Verification items for the finished model (mm, model axes). Face numbers are marked on the shaded views. A direction names the side the tool comes from. Coordinates: 2 decimals unless noted, no trailing zeros. Order: outer loops, then holes, each group sorted by start corner. A loop starts at its lowest first (then second) coordinate and runs counter-clockwise, first axis right, second up. Notation, with made-up numbers: M 72.25,86.25 L 102.25,86.25 A9 ccw 102.25,103.25 Z; hole C 24.25,25 d8. An arc over 180 degrees is marked long. Return JSON: item names as keys, results as strings. Group by question number.
Q1. Section check D-D, the plane y = 18.5. Enter the section's corners in (x, z), then the cut area to 3 significant figures.
Q2. Section check C-C, the plane y = 10.5. Enter the section's corners in (x, z), then the cut area to 3 significant figures.
Q3. Go/stop test with flat-tipped pins: pin 1 Ø5 at (y, z) = (15.5, 9) entering from +X; pin 2 Ø9 at (x, z) = (-19, 7.5) entering from +Y; pin 3 Ø6 at (x, y) = (0, -5) entering from +Z; pin 4 Ø1.8 at (x, y) = (0, -5) entering from +Z. Record where each tip stops, or that it passes through.
Q4. Access from +Z, -Z, +X, -X, +Y, -Y to the whole of each face (thin tool, end or side, straight path). Record for the marked faces 4, 5, 6 and 7.
Q5. Mould release check, pull along Z, two halves, no side actions. Record for the marked faces 1, 2 and 3: pulls with the +Z half, pulls with the -Z half, needs draft (parallel to the pull), parting line crosses it, or undercut.
Q6. Thickness scan on probe 1 along Z at (x, y) = (-6, -26); probe 2 along Z at (x, y) = (19, -10); probe 3 along X at (y, z) = (-27, 10.5). Record the ranges inside material, lowest first.
Q7. Section check B-B, the plane x = 19. Enter the section's corners in (y, z), then the cut area to 3 significant figures.
Q8. Section check A-A, the plane z = 7.5. Count the separate pieces of the cut face and the enclosed holes in it, then the cut area to 3 significant figures.
from build123d import *

# Parameters (mm, degrees)
BOSS_EXTRUDE1_DEPTH = 15
CUT_EXTRUDE1_REACH  = 17
CUT_EXTRUDE2_DEPTH  = 1.5
CUT_EXTRUDE3_REACH  = 15.5
SKETCH4_R           = 1.5
SKETCH5_R           = 2.5
CUT_EXTRUDE4_DEPTH  = 12
SKETCH6_R           = 0.48
BOSS_EXTRUDE2_DEPTH = 1.5
CUT_EXTRUDE5_REACH  = 57
SKETCH7_R           = 2.25
SKETCH8_R           = 5.54
CUT_EXTRUDE6_DEPTH  = 21
CUT_EXTRUDE7_REACH  = 57
SKETCH9_W           = 24
SKETCH9_H           = 7


with BuildPart() as part:
    # Sketch1 → Boss-Extrude1 (new body)
    with BuildSketch(Plane.XY):
        with BuildLine():
            Line((-25, 0), (-25, -30))
            Line((-25, -30), (25, -30))
            Line((25, -30), (25, 0))
            ThreePointArc((25, 0), (0, 25), (-25, 0))
        make_face()
    extrude(amount=BOSS_EXTRUDE1_DEPTH)

    # Sketch2 → Cut-Extrude1 (cut, up to next)
    with BuildSketch(Plane.XY.offset(15), mode=Mode.PRIVATE) as cut_extrude1_sk1:
        with BuildLine():
            Line((-15, -5), (-11.25, -5))
            ThreePointArc((-11.25, -5), (4.305188614, -15.393644741), (7.954951288, 2.954951288))
            Line((7.954951288, 2.954951288), (10.606601718, 5.606601718))
            ThreePointArc((10.606601718, 5.606601718), (5.740251485, -18.858192988), (-15, -5))
        make_face()
    cut_extrude1_tool1 = extrude(cut_extrude1_sk1.sketch, amount=-CUT_EXTRUDE1_REACH, mode=Mode.PRIVATE) & part.part
    add(cut_extrude1_tool1.solids().sort_by_distance((9.559676, 4.001877, 15))[0], mode=Mode.SUBTRACT)

    # Sketch3 → Cut-Extrude2 (cut)
    with BuildSketch(Plane.XY.offset(15)):
        with BuildLine():
            Line((-14.191020378, 1.753883373), (-0.462045472, -1.78301166))
            ThreePointArc((-0.462045472, -1.78301166), (3.054001018, -6.111565466), (-2.421787612, -7.167358937))
            Line((-2.421787612, -7.167358937), (-15.212264853, -1.05196276))
            ThreePointArc((-15.212264853, -1.05196276), (-15.974774553, 0.814342437), (-14.191020378, 1.753883373))
        make_face()
    extrude(amount=-CUT_EXTRUDE2_DEPTH, mode=Mode.SUBTRACT)

    # Sketch4 → Cut-Extrude3 (cut, up to next)
    with BuildSketch(Plane.XY.offset(13.5), mode=Mode.PRIVATE) as cut_extrude3_sk1:
        with Locations((0, -5)):
            Circle(SKETCH4_R)
    cut_extrude3_tool1 = extrude(cut_extrude3_sk1.sketch, amount=-CUT_EXTRUDE3_REACH, mode=Mode.PRIVATE) & part.part
    add(cut_extrude3_tool1.solids().sort_by_distance((0, -5, 13.5))[0], mode=Mode.SUBTRACT)

    # Sketch5 → Cut-Extrude4 (cut)
    with BuildSketch(Plane(origin=(0, 0, 0), x_dir=(-1, 0, 0), z_dir=(0, 0, -1))):
        with Locations((0, -5)):
            Circle(SKETCH5_R)
    extrude(amount=-CUT_EXTRUDE4_DEPTH, mode=Mode.SUBTRACT)

    # Sketch6 → Boss-Extrude2 (add)
    with BuildSketch(Plane.XY.offset(13.5)):
        with Locations((-14.565235622, 0.301312222)):
            Circle(SKETCH6_R)
        with Locations((-12.497911856, -0.451132094)):
            Circle(SKETCH6_R)
        with Locations((-10.430588091, -1.203576409)):
            Circle(SKETCH6_R)
        with Locations((-8.363264325, -1.956020724)):
            Circle(SKETCH6_R)
        with Locations((-6.295940559, -2.70846504)):
            Circle(SKETCH6_R)
        with Locations((-4.228616794, -3.460909355)):
            Circle(SKETCH6_R)
    extrude(amount=BOSS_EXTRUDE2_DEPTH)

    # Sketch7 → Cut-Extrude5 (cut, up to next)
    with BuildSketch(Plane.XZ.offset(30), mode=Mode.PRIVATE) as cut_extrude5_sk1:
        with Locations((-19, 7.5)):
            Circle(SKETCH7_R)
    cut_extrude5_tool1 = extrude(cut_extrude5_sk1.sketch, amount=-CUT_EXTRUDE5_REACH, mode=Mode.PRIVATE) & part.part
    add(cut_extrude5_tool1.solids().sort_by_distance((-19, -30, 7.5))[0], mode=Mode.SUBTRACT)
    # Sketch7 → Cut-Extrude5 (cut, up to next)
    with BuildSketch(Plane.XZ.offset(30), mode=Mode.PRIVATE) as cut_extrude5_sk2:
        with Locations((19, 7.5)):
            Circle(SKETCH7_R)
    cut_extrude5_tool2 = extrude(cut_extrude5_sk2.sketch, amount=-CUT_EXTRUDE5_REACH, mode=Mode.PRIVATE) & part.part
    add(cut_extrude5_tool2.solids().sort_by_distance((19, -30, 7.5))[0], mode=Mode.SUBTRACT)

    # Sketch8 → Cut-Extrude6 (cut)
    with BuildSketch(Plane(origin=(0, 23.467134405, 0), x_dir=(1, 0, 0), z_dir=(0, 1, 0))):
        with Locations((-19, -7.5)):
            Circle(SKETCH8_R)
        with Locations((19, -7.5)):
            Circle(SKETCH8_R)
    extrude(amount=-CUT_EXTRUDE6_DEPTH, mode=Mode.SUBTRACT)

    # Sketch9 → Cut-Extrude7 (cut, up to next)
    with BuildSketch(Plane.XZ.offset(30), mode=Mode.PRIVATE) as cut_extrude7_sk1:
        with Locations((0, 7.5)):
            Rectangle(SKETCH9_W, SKETCH9_H)
    cut_extrude7_tool1 = extrude(cut_extrude7_sk1.sketch, amount=-CUT_EXTRUDE7_REACH, mode=Mode.PRIVATE) & part.part
    add(cut_extrude7_tool1.solids().sort_by_distance((0, -30, 7.5))[0], mode=Mode.SUBTRACT)


solid = part.part
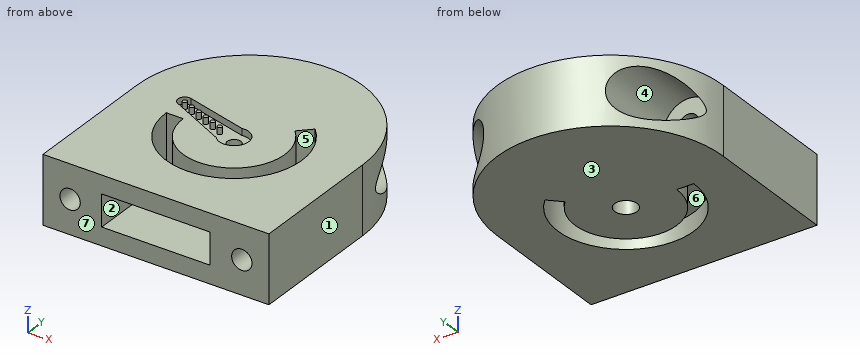
Numbers:
{
 "1": {"outline": "M -16.82,0 L 16.82,0 L 16.82,2.41 A5.54 cw 16.82,12.59 L 16.82,15 L -16.82,15 L -16.82,12.59 A5.54 cw -16.82,2.41 Z", "area": "455 mm2"},
 "2": {"outline": "M -22.69,0 L 22.69,0 L 22.69,3.37 A5.54 cw long 22.69,11.63 L 22.69,15 L -22.69,15 L -22.69,11.63 A5.54 cw long -22.69,3.37 Z", "area": "509 mm2"},
 "3": {"pin 1": "stops at x = 15.17", "pin 2": "stops at y = 2.47", "pin 3": "stops at z = 13.5", "pin 4": "passes through"},
 "4": {"face 4": "+Y", "face 5": "+Z, -Z", "face 6": "-Y", "face 7": "+Z, -Z, +X, -X, -Y"},
 "5": {"face 1": "needs draft", "face 2": "undercut", "face 3": "pulls with the -Z half"},
 "6": {"probe 1": "z = 0 to 4, 11 to 15", "probe 2": "z = 0 to 5.25, 9.75 to 15", "probe 3": "x = -25 to -12, 12 to 25"},
 "7": {"outline": "M -30,0 L 16.25,0 L 16.25,1.96 L 2.47,1.96 L 2.47,5.25 L -30,5.25 Z; M -30,9.75 L 2.47,9.75 L 2.47,13.04 L 16.25,13.04 L 16.25,15 L -30,15 Z", "area": "395 mm2"},
 "8": {"separate pieces": "3", "enclosed holes": "1", "area": "1,410 mm2"}
}
